For this review, use the dimensioned drawing (mm, ordinates from the lowest corner) and the shaded views. A direction names the side the tool comes from. Coordinates: 2 decimals unless noted, no trailing zeros. Order: outer loops, then holes, each group sorted by start corner. A loop starts at its lowest first (then second) coordinate and runs counter-clockwise, first axis right, second up. Notation, with made-up numbers: M 43.25,80.25 L 59.25,80.25 A18 ccw 59.25,88.25 Z; hole C -26,20.5 d9. An arc over 180 degrees is marked long. Answer as CSV lines item,"result". Start each with the question number.
Q1. Consider section D-D on x = 21. Write out the cut boundary in (y, z).
Q2. Consider section A-A on x = 32. Write out the cut boundary in (y, z).
Q3. For P1, Ø7, axis at x = 31, z = 14.5, coming from the +Y side; P2, Ø5, axis at y = 7.5, z = 20, coming from the -X side; P3, Ø1, axis at x = 13, y = 6.5, coming from the +Z side, all flat-tipped, find the tip position at first contact; note any pin that passes through.
Q4. Consider section B-B on z = 12. Write out the cut boundary in (x, y), and give its area (3 significant figures).
Q5. Wall thickness on L1, parallel to Z at x = 32, y = 0.35; L2, parallel to X at y = 0.9, z = 20; L3, parallel to Y at x = 39.5, z = 7.25: over which ranges is each line inside the solid? List them lowest first. Write a range as [from, to].
Q6. Consider section C-C on z = 4.75. Write out the cut boundary in (x, y), and give its area (3 significant figures).
Q7. Machinability: for the marked faces 1 and 2, which of the approach directions +Z, -Z, +X, -X, +Y, -Y give a long, thin tool a straight path to every point of the face, cutting with its end or side? Answer none if there is none.
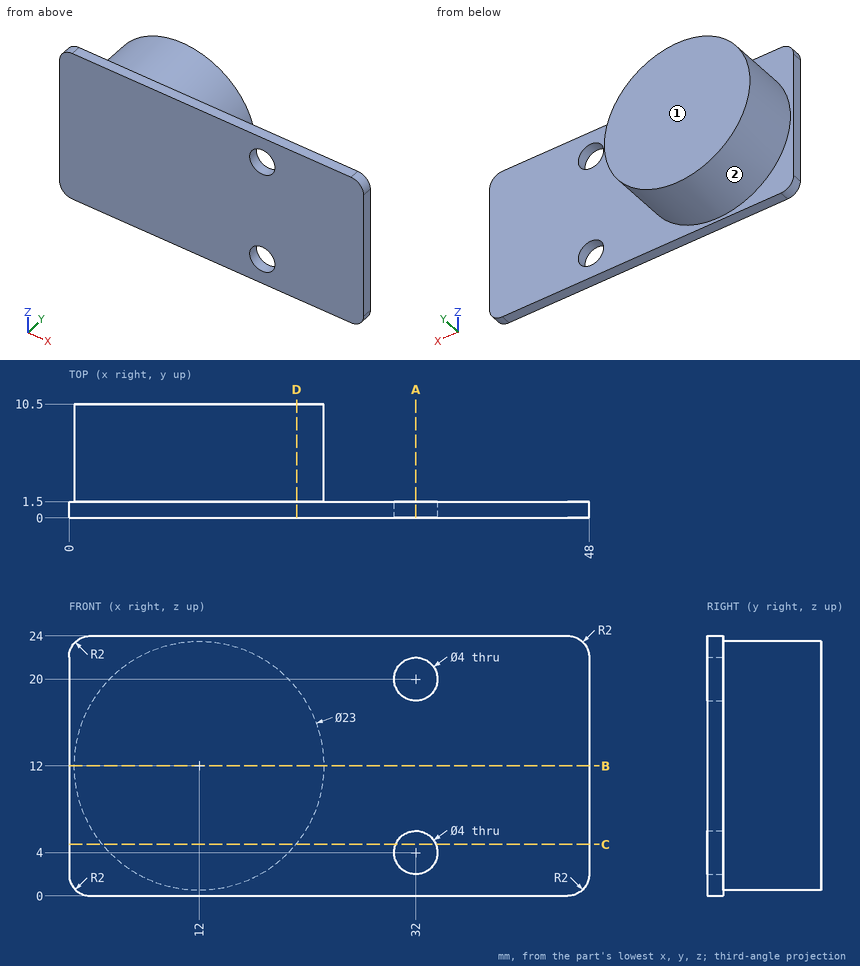
Evaluation:
1,outline,"M 0,0 L 1.5,0 L 1.5,4.84 L 10.5,4.84 L 10.5,19.16 L 1.5,19.16 L 1.5,24 L 0,24 Z"
2,outline,"M 0,0 L 1.5,0 L 1.5,2 L 0,2 Z; M 0,6 L 1.5,6 L 1.5,18 L 0,18 Z; M 0,22 L 1.5,22 L 1.5,24 L 0,24 Z"
3,P1,"stops at y = 1.5"
3,P2,"stops at x = 1.9"
3,P3,"stops at z = 23.49"
4,outline,"M 0,0 L 48,0 L 48,1.5 L 23.5,1.5 L 23.5,10.5 L 0.5,10.5 L 0.5,1.5 L 0,1.5 Z"
4,area,"279 mm²"
5,L1,"z = [0, 2], [6, 18], [22, 24]"
5,L2,"x = [0, 30], [34, 48]"
5,L3,"y = [0, 1.5]"
6,outline,"M 0,0 L 30.15,0 L 30.15,1.5 L 20.93,1.5 L 20.93,10.5 L 3.07,10.5 L 3.07,1.5 L 0,1.5 Z; M 33.85,0 L 48,0 L 48,1.5 L 33.85,1.5 Z"
6,area,"227 mm²"
7,face 1,"+Z, -Z, +X, -X, +Y"
7,face 2,"+Y"
